Autodesk Inventor part; units mm, degrees
ref_plane "YZ Plane" through (0, 0, 0) normal (1, 0, 0) x (0, 1, 0)
ref_plane "XZ Plane" through (0, 0, 0) normal (0, 1, 0) x (-1, 0, 0)
ref_plane "XY Plane" through (0, 0, 0) normal (0, 0, 1) x (1, 0, 0)
sketch "Sketch1" plane through (0, 0, 0) normal (1, 0, 0) x (0, 1, 0)
  circle A0 centre (0, 0) radius 1.75
  circle A1 centre (103.0001, 0.0035) radius 2.5
  circle A2 centre (103.0001, 0.0035) radius 6
  circle A3 centre (0, 0) radius 2.5
  line L0 (102.7964, -5.9931) -> (-0.0849, -2.4986)
  line L1 (102.796, 6) -> (-0.085, 2.4986)
  dimension "d0" = 3.5
  dimension "d1" = 5
  dimension "d2" = 12
  dimension "d3" = 5
extrude "Extrusion1" add sketch "Sketch1" along normal blind 5
properties part number "CoinLockUdløser"
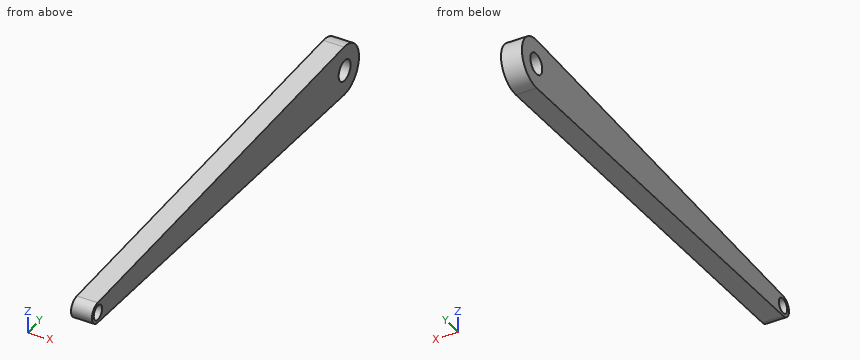
Geometry: final body of the model. Coordinates: model frame, mm. Give positions to 0.01 mm unless a question says otherwise; leave off trailing zeros. Loops run counter-clockwise (first coordinate to the right, second up) from the corner with the lowest first, then second, coordinate; pieces in that order, holes last. Notation, with made-up numbers: (79.5, 8) -> (86.5, 8) arc R15 ccw to (86.5, 27) -> close; hole circle Ø4 at (-13.75, -9). An arc over 180 degrees is marked (long way). Use one line per item in the form item = value.
Item 1: Section query B-B on z = -4.5. Output: boundary loops of the cut face in (x, y).
A:
outline = (0, 58.84) -> (5, 58.84) -> (5, 106.96) -> (0, 106.96) -> close
Item 2: Line query: probe 1 along Z at (x, y) = (2.5, 0); probe 2 along Y at (x, z) = (2.6, -1.5); probe 3 along Y at (x, z) = (2.6, 1). Output: solid intervals per line, ascending.
A:
probe_1 = -2.5 to -1.75, 1.75 to 2.5
probe_2 = -2 to -0.9, 0.9 to 101, 105 to 108.81
probe_3 = -2.29 to -1.44, 1.44 to 100.71, 105.29 to 108.92
Item 3: Section query A-A on x = 0.8. Give the number of separate pieces and of enclosed holes in the cut face, and give its area (3 significant figures).
A:
separate_pieces = 1
enclosed_holes = 2
area = 913 mm^2
Item 4: Section query C-C on y = 78.5. Output: boundary loops of the cut face in (x, z).
A:
outline = (0, -5.17) -> (5, -5.17) -> (5, 5.17) -> (0, 5.17) -> close
Item 5: Pin query (flat end, axial travel): P1, Ø4, axis at y = 103, z = 0, coming from the -X side; P2, Ø1, axis at x = 3, z = 2, coming from the -Y side. Return the tip coordinate at first contact, or that it passes through.
A:
P1 = through
P2 = -2
